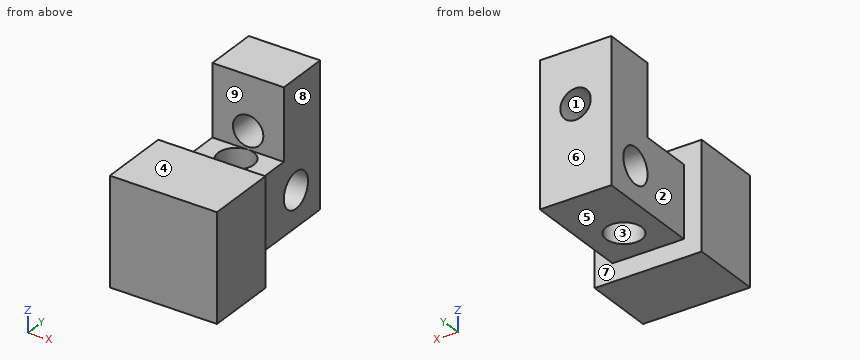
Autodesk Inventor part; units mm, degrees
ref_plane "YZ Plane" through (0, 0, 0) normal (1, 0, 0) x (0, 1, 0)
ref_plane "XZ Plane" through (0, 0, 0) normal (0, 1, 0) x (-1, 0, 0)
ref_plane "XY Plane" through (0, 0, 0) normal (0, 0, 1) x (1, 0, 0)
sketch "Sketch1" plane through (0, 0, 0) normal (0, 0, 1) x (1, 0, 0)
  circle A0 centre (0, 0) radius 1.5875
  line L0 (-3.175, -3.175) -> (3.175, -3.175)
  line L1 (3.175, -3.175) -> (3.175, 6.35)
  line L2 (3.175, 6.35) -> (-3.175, 6.35)
  line L3 (-3.175, 6.35) -> (-3.175, -3.175)
  dimension "d0" = 3.175
  dimension "d2" = 6.35
  dimension "d3" = 3.175
  dimension "d4" = 3.175
  dimension "d5" = 9.525
extrude "Extrusion1" add sketch "Sketch1" along normal blind 6.35
sketch "Sketch2" plane through (3.175, -3.175, 0) normal (1, 0, 0) x (0, 0, -1)
  line L0 (0, 9.525) -> (-6.35, 9.525)
  circle A0 centre (-3.175, 6.35) radius 1.5875
  point P0 (0, 3.175)
  dimension "d8" = 3.175
  dimension "d9" = 3.175
extrude "Extrusion2" cut sketch "Sketch2" against normal up to next
sketch "Sketch3" plane through (0, 0, 6.35) normal (0, 0, 1) x (1, 0, 0)
  line L0 (3.175, -3.175) -> (3.175, 6.35)
  line L1 (-3.175, 6.35) -> (3.175, 6.35)
  line L2 (3.175, 6.35) -> (3.175, 1.5875)
  line L3 (3.175, 1.5875) -> (-3.175, 1.5875)
  line L4 (-3.175, 1.5875) -> (-3.175, 6.35)
  point P0 (3.175, 0)
extrude "Extrusion3" add sketch "Sketch3" along normal blind 6.35
sketch "Sketch4" plane through (-3.175, 6.35, 0) normal (0, 1, 0) x (1, 0, 0)
  circle A0 centre (3.175, -7.9375) radius 1.3525
  line L0 (6.35, 0) -> (0, 0)
  point P0 (3.175, 0)
  dimension "d15" = 2.7051
  dimension "d26" = 7.9375
extrude "Extrusion4" cut sketch "Sketch4" against normal blind 6.35
sketch "Sketch5" plane through (-3.175, -3.175, 0) normal (0, -1, 0) x (1, 0, 0)
  line L0 (0, 0) -> (6.35, 0)
  line L1 (6.35, 0) -> (6.35, 6.35)
  line L2 (0, 6.35) -> (6.35, 6.35)
  line L3 (0, 0) -> (0, 6.35)
  line L4 (-1.5875, 7.9375) -> (7.9375, 7.9375)
  line L5 (7.9375, 7.9375) -> (7.9375, -1.5875)
  line L6 (7.9375, -1.5875) -> (-1.5875, -1.5875)
  line L7 (-1.5875, -1.5875) -> (-1.5875, 7.9375)
  point P0 (3.175, 0)
  dimension "d20" = 1.5875
  dimension "d21" = 1.5875
  dimension "d22" = 1.5875
  dimension "d23" = 1.5875
extrude "Extrusion5" add sketch "Sketch5" along normal blind 6.35 contours L3 L2 L1 L0 | L4 L5 L6 L7
properties part number "quad"
For this review, take the finished solid that the model builds, in its own axes (mm). Face numbers are marked on the shaded views. A direction names the side the tool comes from. Round coordinates to 2 decimals unless told otherwise and drop trailing zeros. One line per question, with ' | ' between items.
Q1. Tool access review of the marked faces 5, 6, 7, 8 and 9: name each direction out of +Z, -Z, +X, -X, +Y, -Y from which nothing blocks a thin tool from reaching the whole face with its end or side.
Taken from the geometry:
face 5: -Z, +X, -X, +Y | face 6: +Z, -Z, +X, -X, +Y | face 7: none | face 8: +Z, -Z, +X, +Y | face 9: +Z, +X, -X
Q2. For pin 1 (1.9 mm diameter, centred on x = -1, y = -7.5, fed in from +Z); pin 2 (1.9 mm diameter, centred on y = 3.175, z = 3.175, fed in from -X); pin 3 (3 mm diameter, centred on x = -0.5, y = 0.5, fed in from -Z); pin 4 (2 mm diameter, centred on y = 3, z = 10.5, fed in from -X) (3 decimals), all flat-tipped, find the tip position at first contact; note any pin that passes through.
Taken from the geometry:
pin 1: stops at z = 7.94 | pin 2: passes through | pin 3: stops at z = 0 | pin 4: stops at x = -3.175
Q3. For line 1 along Z through (x, y) = (1.75, -6.5); line 2 along Y through (x, z) = (1, 2.25) (3 decimals); line 3 along Z through (x, y) = (0, 4.6) (3 decimals), list the stretches that pass through material, from the lowest coordinate up. Write a range as [from, to].
Taken from the geometry:
line 1: z = [-1.59, 7.94] | line 2: y = [-9.525, -1.233], [1.233, 1.885], [4.465, 6.35] | line 3: z = [0, 2.475], [3.875, 6.585], [9.29, 12.7]
Q4. Take a section at A-A (z = 4). State how many separate pieces and enclosed holes the cut face has, and give its area (3 significant figures).
Taken from the geometry:
separate pieces: 2 | enclosed holes: 1 | area: 95.8 mm²
Q5. The part is to be moulded in two halves that separate along X. For the marked faces 1, 2, 3 and 4, say which applies: released by +X, released by -X, zero draft, split by the parting line, or undercut.
Taken from the geometry:
face 1: undercut | face 2: released by -X | face 3: undercut | face 4: zero draft
